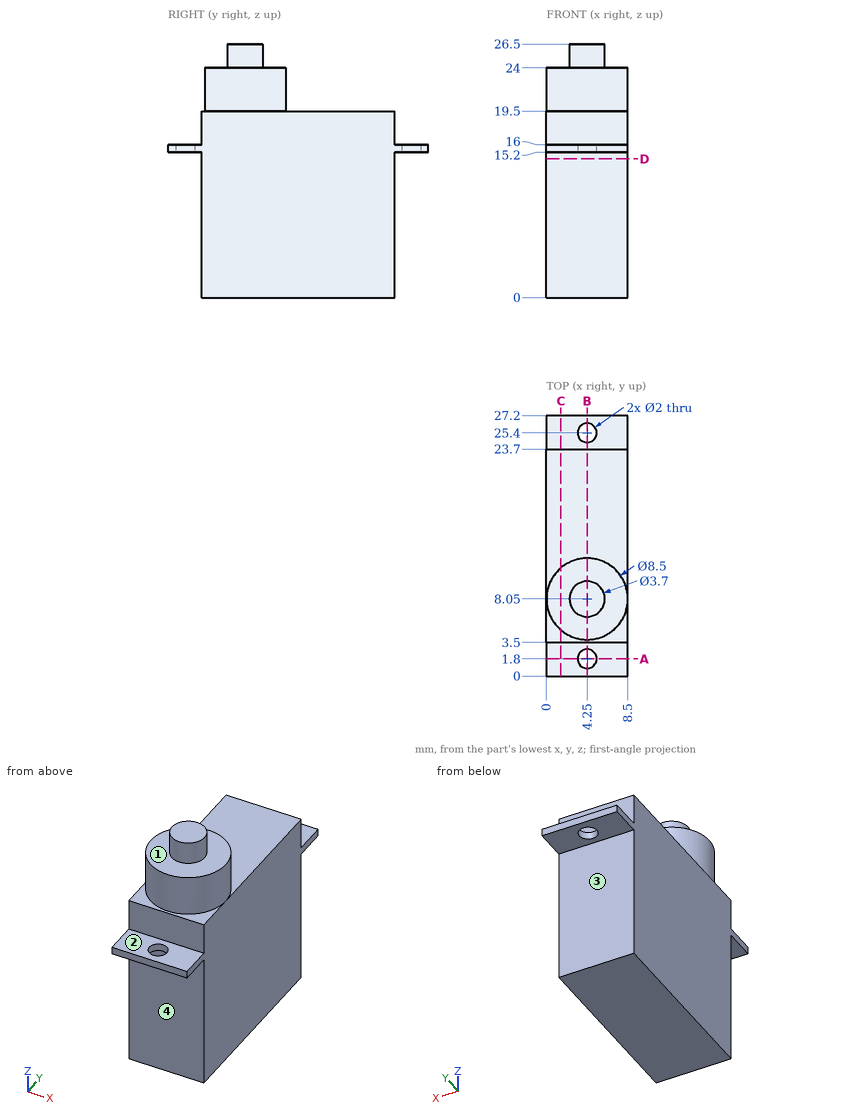
Geometry check sheet. Reference: drawing and pictorial views, mm from the part's lowest x, y, z. A direction names the side the tool comes from. Coordinates: 2 decimals unless noted, no trailing zeros. Write each loop counter-clockwise with the first axis right and the second up, starting at its lowest first coordinate (ties: lowest second). Pieces come first, ordered by that corner, then holes. Notation, with made-up numbers: M 53,48 L 62,48 A36 cw 62,82 Z; hole C -6.75,56 d3. An arc over 180 degrees is marked long. Write item = value, one per line. Start each with the question number.
1. Sectioned sample at D-D (z = 14.5). Record the cut outline in (x, y), then the cut area to 3 significant figures.
2. Tool access check on the marked faces 1, 2, 3 and 4. Record the directions out of +Z, -Z, +X, -X, +Y, -Y that give a thin tool (end or side, any length) a straight path to the whole face; none if there is none.
3. Sectioned sample at C-C (x = 1.5). Record the cut outline in (y, z).
4. Sectioned sample at B-B (x = 4.25). Record the cut outline in (y, z).
5. Thickness scan on probe 1 along Y at (x, z) = (4.25, 15.4); probe 2 along Z at (x, y) = (1, 8.5); probe 3 along Z at (x, y) = (2.5, 25.25). Record the ranges inside material, lowest first.
6. Sectioned sample at A-A (y = 1.8). Record the cut outline in (x, z), then the cut area to 3 significant figures.
7. Go/stop test with flat-tipped pins: pin 1 (2.5 mm diameter, centred on x = 3.5, z = 9.5, fed in from -Y); pin 2 (1 mm diameter, centred on x = 5.5, y = 25.5, fed in from +Z); pin 3 (1.5 mm diameter, centred on x = 3.5, z = 5, fed in from +Y). Record where each tip stops, or that it passes through.
The answers:
q1.outline = M 0,3.5 L 8.5,3.5 L 8.5,23.7 L 0,23.7 Z
q1.area = 172 mm²
q2.face_1 = +Z
q2.face_2 = +Z, +X, -X, -Y
q2.face_3 = -Z, +X, -X, +Y
q2.face_4 = -Z, +X, -X, -Y
q3.outline = M 0,15.2 L 3.5,15.2 L 3.5,0 L 23.7,0 L 23.7,15.2 L 27.2,15.2 L 27.2,16 L 23.7,16 L 23.7,19.5 L 11.29,19.5 L 11.29,24 L 4.81,24 L 4.81,19.5 L 3.5,19.5 L 3.5,16 L 0,16 Z
q4.outline = M 0,15.2 L 0.8,15.2 L 0.8,16 L 0,16 Z; M 2.8,15.2 L 3.5,15.2 L 3.5,0 L 23.7,0 L 23.7,15.2 L 24.4,15.2 L 24.4,16 L 23.7,16 L 23.7,19.5 L 12.3,19.5 L 12.3,24 L 9.9,24 L 9.9,26.5 L 6.2,26.5 L 6.2,24 L 3.8,24 L 3.8,19.5 L 3.5,19.5 L 3.5,16 L 2.8,16 Z; M 26.4,15.2 L 27.2,15.2 L 27.2,16 L 26.4,16 Z
q5.probe_1 = 0 to 0.8, 2.8 to 24.4, 26.4 to 27.2
q5.probe_2 = 0 to 24
q5.probe_3 = 15.2 to 16
q6.outline = M 0,15.2 L 3.25,15.2 L 3.25,16 L 0,16 Z; M 5.25,15.2 L 8.5,15.2 L 8.5,16 L 5.25,16 Z
q6.area = 5.20 mm²
q7.pin_1 = 3.5
q7.pin_2 = 16
q7.pin_3 = 23.7
